```python
from build123d import *

# Parameters (mm, degrees)
SALIENTE_EXTRUIR1_DEPTH  = 170
SALIENTE_EXTRUIR2_DEPTH  = 2.5
CROQUIS4_R               = 4.7625
CORTAR_EXTRUIR1_DEPTH    = 2.5
SALIENTE_EXTRUIR3_DEPTH  = 2.5
SALIENTE_EXTRUIR4_DEPTH  = 80
SALIENTE_EXTRUIR5_DEPTH  = 2.5
CROQUIS8_W               = 140
CROQUIS8_H               = 161
CROQUIS8_W_2             = 80
CROQUIS8_H_2             = 101
SALIENTE_EXTRUIR6_DEPTH  = 2.5
CROQUIS9_R               = 4.7625
CORTAR_EXTRUIR2_DEPTH    = 2.5
CROQUIS10_R              = 61
CORTAR_EXTRUIR3_DEPTH    = 2.5
SALIENTE_EXTRUIR7_START  = 28.5
CROQUIS11_R              = 63.5
CROQUIS11_R_2            = 61
SALIENTE_EXTRUIR7_DEPTH  = 28.5
CROQUIS12_R              = 88
CROQUIS12_R_2            = 61
SALIENTE_EXTRUIR8_DEPTH  = 2.5
CROQUIS13_W              = 175
CROQUIS13_H              = 115
SALIENTE_EXTRUIR9_DEPTH  = 2.5
CROQUIS14_W              = 175
CROQUIS14_H              = 2.5
SALIENTE_EXTRUIR10_DEPTH = 26.5
SALIENTE_EXTRUIR11_DEPTH = 2.5
SALIENTE_EXTRUIR12_DEPTH = 2.5
CROQUIS17_R              = 4.7625
CORTAR_EXTRUIR4_DEPTH    = 2.5
CROQUIS18_R              = 154
SALIENTE_EXTRUIR13_DEPTH = 2.5
CROQUIS19_R              = 3.96875
SALIENTE_EXTRUIR14_DEPTH = 16
MATRIZC1_COUNT           = 6
CROQUIS20_R              = 3.96875
SALIENTE_EXTRUIR15_DEPTH = 7
MATRIZC3_COUNT           = 6


with BuildPart() as part:
    # Croquis1 → Saliente-Extruir1 (new body)
    with BuildSketch(Plane.XY):
        Polygon((0, 0), (29, 0), (75, 197), (235, 197), (281, 0), (310, 0), (310, 2.5), (282.983493442, 2.5), (236.983493442, 199.5), (73.016506558, 199.5), (27.016506558, 2.5), (0, 2.5), align=None)
    extrude(amount=SALIENTE_EXTRUIR1_DEPTH)

    # Croquis2 → Saliente-Extruir2 (add)
    with BuildSketch(Plane.XY.offset(170)):
        Polygon((29, 0), (281, 0), (269.286291687, 50.165229078), (235, 197), (75, 197), (40.713708313, 50.165229078), align=None)
        Polygon((243.652375223, 50), (66.347624777, 50), (94.834934422, 172), (215.165065578, 172), align=None, mode=Mode.SUBTRACT)
    extrude(amount=-SALIENTE_EXTRUIR2_DEPTH)

    # Croquis4 → Cortar-Extruir1 (cut)
    with BuildSketch(Plane(origin=(0, 2.5, 0), x_dir=(1, 0, 0), z_dir=(0, 1, 0))):
        with Locations(Location((13.508253279, -30, 0), (0, 0, 270))):
            Circle(CROQUIS4_R)
        with Locations(Location((13.508253279, -140, 0), (0, 0, 270))):
            Circle(CROQUIS4_R)
        with Locations(Location((296.491746721, -140, 0), (0, 0, 90))):
            Circle(CROQUIS4_R)
        with Locations(Location((296.491746721, -30, 0), (0, 0, 90))):
            Circle(CROQUIS4_R)
    extrude(amount=-CORTAR_EXTRUIR1_DEPTH, mode=Mode.SUBTRACT)

    # Croquis5 → Saliente-Extruir3 (add)
    with BuildSketch(Plane(origin=(0, 0, 0), x_dir=(-1, 0, 0), z_dir=(0, 0, -1))):
        with BuildLine():
            Line((0, 30), (40, 30))
            Line((40, 30), (40, 135))
            Line((40, 135), (-10, 135))
            ThreePointArc((-10, 135), (13.653759217, 342.621891967), (-152, 470))
            ThreePointArc((-152, 470), (-372, 250), (-152, 30))
            Line((-152, 30), (0, 30))
        make_face()
    extrude(amount=SALIENTE_EXTRUIR3_DEPTH)

    # Croquis6 → Saliente-Extruir4 (add)
    with BuildSketch(Plane(origin=(0, 0, -2.5), x_dir=(-1, 0, 0), z_dir=(0, 0, -1))):
        with BuildLine():
            Line((-10, 135), (40, 135))
            Line((40, 135), (40, 133))
            Line((40, 133), (38, 133))
            Line((38, 133), (-13.968512136, 133))
            ThreePointArc((-13.968512136, 133), (12.60152192, 339.954109112), (-152.141403753, 467.99995414))
            ThreePointArc((-152.141403753, 467.99995414), (-369.999988535, 249.92929812), (-152, 32))
            Line((-152, 32), (38, 32))
            Line((38, 32), (40, 32))
            Line((40, 32), (40, 30))
            Line((40, 30), (-152, 30))
            ThreePointArc((-152, 30), (-372, 250), (-152, 470))
            ThreePointArc((-152, 470), (13.653759217, 342.621891967), (-10, 135))
        make_face()
    extrude(amount=SALIENTE_EXTRUIR4_DEPTH)

    # Croquis7 → Saliente-Extruir5 (add)
    with BuildSketch(Plane(origin=(0, 0, -82.5), x_dir=(-1, 0, 0), z_dir=(0, 0, -1))):
        with BuildLine():
            Line((-10, 135), (40, 135))
            Line((40, 135), (40, 30))
            Line((40, 30), (-152, 30))
            ThreePointArc((-152, 30), (-372, 250), (-152, 470))
            ThreePointArc((-152, 470), (13.653759217, 342.621891967), (-10, 135))
        make_face()
    extrude(amount=SALIENTE_EXTRUIR5_DEPTH)

    # Croquis8 → Saliente-Extruir6 (add)
    with BuildSketch(Plane.ZY.offset(40)):
        with Locations((-42.5, 82.5)):
            Rectangle(CROQUIS8_W, CROQUIS8_H)
        with Locations((-42.5, 82.5)):
            Rectangle(CROQUIS8_W_2, CROQUIS8_H_2, mode=Mode.SUBTRACT)
    extrude(amount=-SALIENTE_EXTRUIR6_DEPTH)

    # Croquis9 → Cortar-Extruir2 (cut)
    with BuildSketch(Plane.ZY.offset(40)):
        with Locations((-42.5, 148)):
            Circle(CROQUIS9_R)
        with Locations((-97.5, 113)):
            Circle(CROQUIS9_R)
        with Locations((12.5, 113)):
            Circle(CROQUIS9_R)
        with Locations(Location((12.5, 52, 0), (0, 0, 180))):
            Circle(CROQUIS9_R)
        with Locations(Location((-97.5, 52, 0), (0, 0, 180))):
            Circle(CROQUIS9_R)
        with Locations(Location((-42.5, 17, 0), (0, 0, 180))):
            Circle(CROQUIS9_R)
    extrude(amount=-CORTAR_EXTRUIR2_DEPTH, mode=Mode.SUBTRACT)

    # Croquis10 → Cortar-Extruir3 (cut)
    with BuildSketch(Plane(origin=(0, 0, -85), x_dir=(-1, 0, 0), z_dir=(0, 0, -1))):
        with Locations((-155, 279.5)):
            Circle(CROQUIS10_R)
    extrude(amount=-CORTAR_EXTRUIR3_DEPTH, mode=Mode.SUBTRACT)

    # Croquis11 → Saliente-Extruir7 (add)
    with BuildSketch(Plane(origin=(0, 0, -85), x_dir=(-1, 0, 0), z_dir=(0, 0, -1)).offset(SALIENTE_EXTRUIR7_START)):
        with Locations(Location((-155, 279.5, 0), (0, 0, 180))):
            Circle(CROQUIS11_R)
        with Locations((-155, 279.5)):
            Circle(CROQUIS11_R_2, mode=Mode.SUBTRACT)
    extrude(amount=-SALIENTE_EXTRUIR7_DEPTH)

    # Croquis12 → Saliente-Extruir8 (add)
    with BuildSketch(Plane(origin=(0, 0, -113.5), x_dir=(-1, 0, 0), z_dir=(0, 0, -1))):
        with Locations((-155, 279.5)):
            Circle(CROQUIS12_R)
        with Locations((-155, 279.5)):
            Circle(CROQUIS12_R_2, mode=Mode.SUBTRACT)
    extrude(amount=-SALIENTE_EXTRUIR8_DEPTH)

    # Croquis13 → Saliente-Extruir9 (add)
    with BuildSketch(Plane(origin=(0, 0, -85), x_dir=(-1, 0, 0), z_dir=(0, 0, -1))):
        with Locations((-155, 57.5)):
            Rectangle(CROQUIS13_W, CROQUIS13_H)
    extrude(amount=SALIENTE_EXTRUIR9_DEPTH)

    # Croquis14 → Saliente-Extruir10 (add)
    with BuildSketch(Plane(origin=(0, 0, -87.5), x_dir=(-1, 0, 0), z_dir=(0, 0, -1))):
        with Locations((-155, 1.25)):
            Rectangle(CROQUIS14_W, CROQUIS14_H)
    extrude(amount=SALIENTE_EXTRUIR10_DEPTH)

    # Croquis15 → Saliente-Extruir11 (add)
    with BuildSketch(Plane.ZY.offset(-67.5)):
        Polygon((-114, 2.5), (-87.5, 115), (-85, 115), (-85, 0), (-114, 0), align=None)
    extrude(amount=-SALIENTE_EXTRUIR11_DEPTH)

    # Croquis16 → Saliente-Extruir12 (add)
    with BuildSketch(Plane(origin=(242.5, 0, 0), x_dir=(0, 0, -1), z_dir=(1, 0, 0))):
        Polygon((114, 2.5), (87.5, 115), (85, 115), (85, 0), (114, 0), align=None)
    extrude(amount=-SALIENTE_EXTRUIR12_DEPTH)

    # Croquis17 → Cortar-Extruir4 (cut)
    with BuildSketch(Plane.XZ):
        with Locations(Location((198.5, -100.75, 0), (0, 0, 270))):
            Circle(CROQUIS17_R)
        with Locations(Location((111.5, -100.75, 0), (0, 0, 270))):
            Circle(CROQUIS17_R)
    extrude(amount=-CORTAR_EXTRUIR4_DEPTH, mode=Mode.SUBTRACT)

    # Croquis18 → Saliente-Extruir13 (add)
    with BuildSketch(Plane(origin=(0, 0, -85), x_dir=(-1, 0, 0), z_dir=(0, 0, -1))):
        with Locations(Location((-155, 279.5, 0), (0, 0, 180))):
            Circle(CROQUIS18_R)
    extrude(amount=SALIENTE_EXTRUIR13_DEPTH)

    # Croquis19 → Saliente-Extruir14 (add)
    with BuildSketch(Plane(origin=(0, 0, -87.5), x_dir=(-1, 0, 0), z_dir=(0, 0, -1))):
        with Locations((-13, 279.5)):
            Circle(CROQUIS19_R)
    saliente_extruir14 = extrude(amount=SALIENTE_EXTRUIR14_DEPTH)

    # MatrizC1: Saliente-Extruir14 ×6 about axis
    matrizc1_axis = Axis((155, 279.5, 0), (0, 0, 1))
    for i in range(1, MATRIZC1_COUNT):
        add(saliente_extruir14.rotate(matrizc1_axis, i * 360 / MATRIZC1_COUNT))

    # Croquis20 → Saliente-Extruir15 (add)
    with BuildSketch(Plane(origin=(0, 0, -87.5), x_dir=(-1, 0, 0), z_dir=(0, 0, -1))):
        Polygon((-6.07179677, 279.5), (-9.535898385, 285.5), (-16.464101615, 285.5), (-19.92820323, 279.5), (-16.464101615, 273.5), (-9.535898385, 273.5), align=None)
        with Locations((-13, 279.5)):
            Circle(CROQUIS20_R, mode=Mode.SUBTRACT)
    saliente_extruir15 = extrude(amount=SALIENTE_EXTRUIR15_DEPTH)

    # MatrizC3: Saliente-Extruir15 ×6 about axis
    matrizc3_axis = Axis((155, 279.5, 0), (0, 0, 1))
    for i in range(1, MATRIZC3_COUNT):
        add(saliente_extruir15.rotate(matrizc3_axis, i * 360 / MATRIZC3_COUNT))


solid = part.part
```
Check sheet for the modelled part. Datum: model origin and axes. Units: mm. A direction names the side the tool comes from. Round coordinates to 2 decimals unless told otherwise and drop trailing zeros. Order: outer loops, then holes, each group sorted by start corner. A loop starts at its lowest first (then second) coordinate and runs counter-clockwise, first axis right, second up.
1) Section check B-B (x = 135.5). Give the number of separate pieces and of enclosed holes in the cut face, and give its area (3 significant figures).
2) Section check D-D (x = 343.5). Record the boundary of the cut face in (y, z), and give its area (3 significant figures).
3) Mould release check, pull along X, two halves, no side actions. Record for faces 6 (the flat face through (80.392, 110.146, 168.768)), 7 (the flat face through (129, 221, -111)), 8 (the cylindrical face through (71.064, 305.933, -112.268)), 9 (the flat face through (242.5, 46, -96)): +X half, -X half, draft (parallel to the pull), parting line (faces both ways), or undercut.
4) Section check A-A (y = 440.5). Record the boundary of the cut face in (x, z).
5) Section check C-C (z = -74.5). Record the boundary of the cut face in (x, y).
6) Tool access check on faces 1 (the flat face through (156, 199.5, 84)), 2 (the flat face through (156, 14, -85)), 3 (the cylindrical face through (369.95, 254.72, -41.94)), 4 (the flat face through (297, 2.5, 84)), 5 (the flat face through (156, 2.5, -101)). Record the directions out of +Z, -Z, +X, -X, +Y, -Y that give a thin tool (end or side, any length) a straight path to the whole face; none if there is none.
7) Go/stop test with flat-tipped pins: pin 1 Ø3 at (y, z) = (71, -20) entering from +X; pin 2 Ø0.8 at (y, z) = (2, 65.5) entering from -X; pin 3 Ø6 at (y, z) = (126, 27) entering from +X. Record where each tip stops, or that it passes through.
8) Scan lines: line 1 (Y direction, x = 155, z = -95.5); line 2 (Z direction, x = -38, y = 52); line 3 (Z direction, x = 190, y = 213). Record each from-to range of solid material in increasing order.
Result:
1. separate pieces: 2
1. enclosed holes: 1
1. area: 4,210 mm2
2. outline: (141.71, -85) - (358.29, -85) - (358.29, 0) - (141.71, 0) - close; hole (145.83, -82.5) - (354.17, -82.5) - (354.17, -2.5) - (145.83, -2.5) - close
2. area: 1,740 mm2
3. face 6: undercut
3. face 7: draft
3. face 8: parting line
3. face 9: +X half
4. outline: (70.4, -85) - (262.04, -85) - (262.04, 0) - (70.4, 0) - close; hole (74.26, -82.5) - (257.99, -82.5) - (257.99, -2.5) - (74.26, -2.5) - close
5. outline: (-40, 2) - (-37.5, 2) - (-37.5, 30) - (152, 30) arc R220 ccw to (152, 470) arc R212.37 ccw to (10, 135) - (-37.5, 135) - (-37.5, 163) - (-40, 163) - (-40, 133) - (13.97, 133) arc R210.37 cw to (152.14, 468) arc R218 cw to (152, 32) - (-40, 32) - close
6. face 1: +Z, +X, -X, +Y
6. face 2: +X, -Y
6. face 3: none
6. face 4: +Z, -Z, +X, +Y
6. face 5: -Z
7. pin 1: stops at x = 281.98
7. pin 2: stops at x = 0
7. pin 3: stops at x = 254.85
8. line 1: y = 0 to 2.5, 216 to 218.5, 340.5 to 343
8. line 2: z = -112.5 to -102.26, -92.74 to -82.5, -2.5 to 7.74, 17.26 to 27.5
8. line 3: z = -113.5 to -111, -87.5 to -82.5, -2.5 to 0
